from build123d import *

# Parameters (mm, degrees)
SKETCH_1_R      = 2.1
EXTRUDE_1_DEPTH = 20
FILLET_1_R      = 1
FILLET_2_R      = 0.3


with BuildPart() as part:
    # Эскиз1 → Бобышка-Вытянуть1 (new body)
    with BuildSketch(Plane.XY):
        Polygon((-10, 10), (-4.4, 10), (-2.6, 8.2), (-5.499339828, 8.2), (-5.499339828, 6.56), (-2.84, 3.900660172), (-0.5, 3.900660172), (0, 3.400660172), (0.5, 3.900660172), (2.84, 3.900660172), (5.499339828, 6.56), (5.499339828, 8.2), (2.6, 8.2), (4.4, 10), (10, 10), (10, 4.4), (8.2, 2.6), (8.2, 5.499339828), (6.56, 5.499339828), (3.900660172, 2.84), (3.900660172, 0.5), (3.400660172, 0), (3.900660172, -0.5), (3.900660172, -2.84), (6.56, -5.499339828), (8.2, -5.499339828), (8.2, -2.6), (10, -4.4), (10, -10), (4.4, -10), (2.6, -8.2), (5.499339828, -8.2), (5.499339828, -6.56), (2.84, -3.900660172), (0.5, -3.900660172), (0, -3.400660172), (-0.5, -3.900660172), (-2.84, -3.900660172), (-5.499339828, -6.56), (-5.499339828, -8.2), (-2.6, -8.2), (-4.4, -10), (-10, -10), (-10, -4.4), (-8.2, -2.6), (-8.2, -5.499339828), (-6.56, -5.499339828), (-3.900660172, -2.84), (-3.900660172, -0.5), (-3.400660172, 0), (-3.900660172, 0.5), (-3.900660172, 2.84), (-6.56, 5.499339828), (-8.2, 5.499339828), (-8.2, 2.6), (-10, 4.4), align=None)
        Circle(SKETCH_1_R, mode=Mode.SUBTRACT)
    extrude(amount=EXTRUDE_1_DEPTH)

    # Скругление1
    fillet_1_edges = [part.edges().sort_by_distance(p)[0] for p in [
        (-10, 10, 10),
        (10, 10, 10),
        (10, -10, 10),
        (-10, -10, 10),
    ]]
    fillet(fillet_1_edges, radius=FILLET_1_R)

    # Скругление2
    fillet_2_edges = [part.edges().sort_by_distance(p)[0] for p in [
        (-4.4, 10, 10),
        (-2.6, 8.2, 10),
        (-5.499339828, 8.2, 10),
        (-5.499339828, 6.56, 10),
        (-2.84, 3.900660172, 10),
        (-0.5, 3.900660172, 10),
        (0.5, 3.900660172, 10),
        (2.84, 3.900660172, 10),
        (5.499339828, 6.56, 10),
        (5.499339828, 8.2, 10),
        (2.6, 8.2, 10),
        (4.4, 10, 10),
        (10, 4.4, 10),
        (8.2, 2.6, 10),
        (8.2, 5.499339828, 10),
        (6.56, 5.499339828, 10),
        (3.900660172, 2.84, 10),
        (3.900660172, 0.5, 10),
        (3.900660172, -0.5, 10),
        (3.900660172, -2.84, 10),
        (6.56, -5.499339828, 10),
        (8.2, -5.499339828, 10),
        (8.2, -2.6, 10),
        (10, -4.4, 10),
        (4.4, -10, 10),
        (2.6, -8.2, 10),
        (5.499339828, -8.2, 10),
        (5.499339828, -6.56, 10),
        (2.84, -3.900660172, 10),
        (0.5, -3.900660172, 10),
        (-0.5, -3.900660172, 10),
        (-2.84, -3.900660172, 10),
        (-5.499339828, -6.56, 10),
        (-5.499339828, -8.2, 10),
        (-2.6, -8.2, 10),
        (-4.4, -10, 10),
        (-10, -4.4, 10),
        (-8.2, -2.6, 10),
        (-8.2, -5.499339828, 10),
        (-6.56, -5.499339828, 10),
        (-3.900660172, -2.84, 10),
        (-3.900660172, -0.5, 10),
        (-3.900660172, 0.5, 10),
        (-3.900660172, 2.84, 10),
        (-6.56, 5.499339828, 10),
        (-8.2, 5.499339828, 10),
        (-8.2, 2.6, 10),
    ]]
    fillet(fillet_2_edges, radius=FILLET_2_R)


solid = part.part
Design review of the part built by this model. Coordinates are the model's own, in mm. A direction names the side the tool comes from. Coordinates: 2 decimals unless noted, no trailing zeros. Write each loop counter-clockwise with the first axis right and the second up, starting at its lowest first coordinate (ties: lowest second). Pieces come first, ordered by that corner, then holes. Notation, with made-up numbers: (-0.75, 0.5) - (42.25, 0.5) arc R18 cw to (42.25, 11.5) - close; hole circle Ø7 at (-27.5, 35). An arc over 180 degrees is marked (long way). Use one line per item in the form item = value.
Q1. For probe 1 along X at (y, z) = (-4.75, 7); probe 2 along X at (y, z) = (-3.75, 19); probe 3 along X at (y, z) = (9, 18), list the stretches that pass through material, from the lowest coordinate up.
Taken from the geometry:
probe_1 = -10 to -8.2, -5.81 to -3.69, 3.69 to 5.81, 8.2 to 10
probe_2 = -9.35 to -8.2, -4.81 to -0.35, 0.35 to 4.81, 8.2 to 9.35
probe_3 = -10 to -3.4, 3.4 to 10
Q2. Machinability: for faces 5 (the flat face through (-5.21, 4.15, 9.86)), 6 (the flat face through (7, 10, 10)), 7 (the flat face through (3.7, 9.3, 9.9)), 8 (the flat face through (3.901, 2, 10)), 9 (the flat face through (-3.901, -2, 10)), which of the approach directions +Z, -Z, +X, -X, +Y, -Y give a long, thin tool a straight path to every point of the face, cutting with its end or side? Answer none if there is none.
Taken from the geometry:
face_5 = +Z, -Z
face_6 = +Z, -Z, +X, -X, +Y
face_7 = +Z, -Z, +Y
face_8 = +Z, -Z, +X
face_9 = +Z, -Z, -X
Q3. The part is to be moulded in two halves that separate along Y. For faces 1 (the cylindrical face through (-9.699, 9.715, 10.14)), 2 (the flat face through (-4, 8.2, 10)), 3 (the flat face through (10, -7, 10)), 4 (the flat face through (4.19, -5.25, 9.86)), say which applies: +Y half, -Y half, draft (parallel to the pull), parting line (faces both ways), or undercut.
Taken from the geometry:
face_1 = +Y half
face_2 = undercut
face_3 = draft
face_4 = undercut
Q4. Consider section A-A (y = -1). Write out the cut boundary in (x, z), plus the area to 3 significant figures.
Taken from the geometry:
outline = (-3.9, 0) - (-1.85, 0) - (-1.85, 20) - (-3.9, 20) - close; (1.85, 0) - (3.9, 0) - (3.9, 20) - (1.85, 20) - close
area = 82.2 mm^2
Q5. Insertion check: pin 1 Ø0.9 at (y, z) = (-4, 9.5) entering from -X; pin 2 Ø0.9 at (x, z) = (-4, 12.5) entering from +Y; pin 3 Ø1 at (y, z) = (3, 4) entering from +X. Each pin has a flat end and moves straight along its axis. Give the tip position at first contact, or say it passes through.
Taken from the geometry:
pin_1 = -9.99
pin_2 = 9.99
pin_3 = 9.1
